```python
from build123d import *

# Parameters (mm, degrees)
F0_W        = 9
F0_H        = 111.76
F1_DEPTH    = 2
F2_R        = 5.08
F3_T1_DEPTH = 26.7289304257
F4_R        = 5.08
F5_T1_DEPTH = 26.7289304257


# Not quite as in the source:
# - a fillet or chamfer that OpenCascade refuses, or shapes differently, is made with other operations: its cross-section is extruded or revolved along the edge and cut away or added


with BuildPart() as f1:
    # F0 (on Front) → F1 (new body)
    with BuildSketch(Plane.XZ):
        with Locations((-4.5, 7.7518613339)):
            Rectangle(F0_W, F0_H)
    extrude(amount=F1_DEPTH)

    # F2
    f2_edges = [f1.edges().sort_by_distance(p)[0] for p in [
        (-9, -1, 63.631861),
    ]]
    fillet(f2_edges, radius=F2_R)

    # F3: fillet of radius 5.08 on 1 edges, made by hand

    # F3_s2 → F3_t1 (cut)
    with BuildSketch(Plane.XZ.offset(-12.3644652129)):
        with BuildLine():
            ThreePointArc((-3.92, 63.6318613339), (-1.0988443889, 61.8415149962), (0, 58.6860752487))
            Line((0, 58.6860752487), (0, 63.6318613339))
            Line((0, 63.6318613339), (-3.92, 63.6318613339))
        make_face()
    extrude(amount=F3_T1_DEPTH, mode=Mode.SUBTRACT)

    # F4
    f4_edges = [f1.edges().sort_by_distance(p)[0] for p in [
        (-9, -1, -48.128139),
    ]]
    fillet(f4_edges, radius=F4_R)

    # F5: fillet of radius 5.08 on 1 edges, made by hand

    # F5_s2 → F5_t1 (cut)
    with BuildSketch(Plane.XZ.offset(-12.3644652129)):
        with BuildLine():
            ThreePointArc((-3.92, -48.1281386661), (-1.0988443889, -46.3377923285), (0, -43.182352581))
            Line((0, -43.182352581), (0, -48.1281386661))
            Line((0, -48.1281386661), (-3.92, -48.1281386661))
        make_face()
    extrude(amount=F5_T1_DEPTH, mode=Mode.SUBTRACT)


solid = f1.part
```
Geometry: final body of the model. Coordinates: model frame, mm. Round coordinates to 2 decimals unless told otherwise and drop trailing zeros. Order: outer loops, then holes, each group sorted by start corner. A loop starts at its lowest first (then second) coordinate and runs counter-clockwise, first axis right, second up. Notation, with made-up numbers: (80, 83.5) - (93, 83.5) arc R16 ccw to (93, 103.5) - close; hole circle Ø9 at (32, 59.25). An arc over 180 degrees is marked (long way). Use CSV: the item, a comma, the result in double quotes. Start each with the question number.
Q1. Material intervals for line 1 along Z through (x, y) = (-7, -1.4); line 2 along Z through (x, y) = (-5.25, -1.3), sorted ascending. Write a range as from..to.
Q2. Section query B-B (x = -1.75). Return loops of the section in (y, z), and give its area (3 significant figures).
Q3. Section query A-A (y = -1.6). Return loops of the section in (x, z), and give its area (3 significant figures).
Result set:
1,line 1,"z = -47.09..62.59"
1,line 2,"z = -47.95..63.45"
2,outline,"(-2, -47.02) - (0, -47.02) - (0, 62.52) - (-2, 62.52) - close"
2,area,"219 mm2"
3,outline,"(-9, -43.05) arc R5.08 ccw to (-3.92, -48.13) arc R5.08 ccw to (0, -43.18) - (0, 58.69) arc R5.08 ccw to (-3.92, 63.63) arc R5.08 ccw to (-9, 58.55) - close"
3,area,"985 mm2"
